from build123d import *

# Parameters (mm, degrees)
F0_R     = 22.198621642
F1_DEPTH = 63.5
F2_R     = 17.4774608617
F3_DEPTH = 7.62
F4_T     = -2.54


with BuildPart() as f1:
    # F0 (on Top) → F1 (new body)
    with BuildSketch(Plane.XY):
        with Locations((-14.8193594068, 37.2680351138)):
            Circle(F0_R)
    extrude(amount=F1_DEPTH)

    # F2 (on face) → F3 (join)
    with BuildSketch(Plane(origin=(0, 0, 0), x_dir=(1, 0, 0), z_dir=(0, 0, -1))):
        with Locations((-14.8193594068, -37.2680351138)):
            Circle(F2_R)
    extrude(amount=F3_DEPTH)

    # F4
    f4_openings = [f1.faces().sort_by_distance(p)[0] for p in [
        (-14.819359, 37.268035, 63.5),
    ]]
    offset(amount=F4_T, openings=f4_openings, kind=Kind.INTERSECTION)


solid = f1.part
The listing builds one solid part. Answer for the finished solid, in the listing's coordinates (mm). A direction names the side the tool comes from. Give positions to 0.01 mm unless a question says otherwise; leave off trailing zeros. Write each loop counter-clockwise with the first axis right and the second up, starting at its lowest first coordinate (ties: lowest second). Pieces come first, ordered by that corner, then holes.
1) Section A-A (x = -8) is taken. Write down the section's boundary in (y, z), and give its area (3 significant figures).
2) For a pull along Y with two mould halves and no side action, classify faces 1 (the face through (-15, 37, -7.62)), 2 (the face through (6.354, 43.936, 31.306)), 3 (the face through (-29.742, 36.611, -1.217)) as pulls with the +Y half, pulls with the -Y half, needs draft (parallel to the pull), parting line crosses it, or undercut.
3) Find the intervals of material crossed by L1, parallel to Y at x = -14.5, z = 36; L2, parallel to Z at x = -27, y = 43.5; L3, parallel to Y at x = -32.5, z = 42, in increasing order.
4) A tool of negligible diameter and unlimited length cuts with its end or side. For faces 4 (the face through (-6.75, 52.77, -3.76)), 5 (the face through (-23, 19, 63.5)), 6 (the face through (-15, 37, -5.08)), from which of +Z, -Z, +X, -X, +Y, -Y can it reach the whole face along a straight path? Write none if from no direction.
5) Section B-B (y = 39) is taken. Write down the section's boundary in (x, z).
6) Given P1, Ø12, axis at x = -21, z = 21, coming from the +Y side; P2, Ø1.5, axis at y = 31.5, z = 31, coming from the -X side; P3, Ø19.5, axis at x = -13, y = 42.5, coming from the +Z side, each flat-ended and moving along its own axis, determine where each tip first touches the part or whether it passes through.
7) Section C-C (z = 38.5) is taken. Write down the section's boundary in (x, y).
Response:
1. outline: (16.14, 0) - (21.18, 0) - (21.18, -7.62) - (53.36, -7.62) - (53.36, 0) - (58.39, 0) - (58.39, 63.5) - (55.71, 63.5) - (55.71, 2.54) - (50.56, 2.54) - (50.56, -5.08) - (23.98, -5.08) - (23.98, 2.54) - (18.83, 2.54) - (18.83, 63.5) - (16.14, 63.5) - close
1. area: 478 mm2
2. face 1: needs draft
2. face 2: parting line crosses it
2. face 3: undercut
3. L1: y = 15.07 to 17.61, 56.92 to 59.46
3. L2: z = -7.62 to -5.08
3. L3: y = 23.85 to 28.67, 45.86 to 50.69
4. face 4: -Z
4. face 5: +Z, +X, -X, +Y, -Y
4. face 6: +Z
5. outline: (-36.95, 0) - (-32.21, 0) - (-32.21, -7.62) - (2.57, -7.62) - (2.57, 0) - (7.31, 0) - (7.31, 63.5) - (4.76, 63.5) - (4.76, 2.54) - (0.02, 2.54) - (0.02, -5.08) - (-29.66, -5.08) - (-29.66, 2.54) - (-34.4, 2.54) - (-34.4, 63.5) - (-36.95, 63.5) - close
6. P1: stops at y = 59.47
6. P2: stops at x = -36.44
6. P3: stops at z = 2.54
7. outline: circle Ø44.4 at (-14.82, 37.27); hole circle Ø39.32 at (-14.82, 37.27)
